Design review of the part built by this model. Coordinates are the model's own, in mm. Face numbers are marked on the shaded views. A direction names the side the tool comes from. Give positions to 0.01 mm unless a question says otherwise; leave off trailing zeros. Write each loop counter-clockwise with the first axis right and the second up, starting at its lowest first coordinate (ties: lowest second). Pieces come first, ordered by that corner, then holes. Notation, with made-up numbers: M 78,-21.5 L 129,-21.5 A4 ccw 129,-16.5 Z; hole C 76.5,-6 d7. An arc over 180 degrees is marked long. Answer in a Markdown table with one row per item.
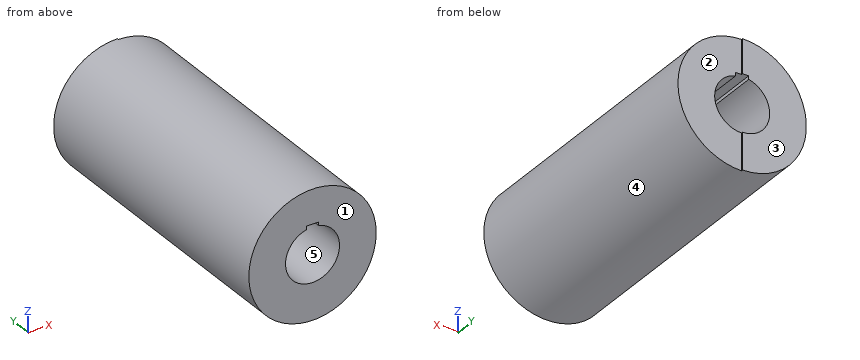
```python
from build123d import *

# Parameters (mm, degrees)
F1_R     = 210
F1_R_2   = 89
F2_DEPTH = 960
F3_W     = 40
F3_H     = 35.969428
F4_DEPTH = 1035
F6_DEPTH = 5


with BuildPart() as f2:
    # F1 (on face) → F2 (new body)
    with BuildSketch(Plane.XZ):
        Circle(F1_R)
        Circle(F1_R_2, mode=Mode.SUBTRACT)
    extrude(amount=F2_DEPTH)

    # F3 (on face) → F4 (cut)
    with BuildSketch(Plane.XZ.offset(960)):
        with Locations((0, 80.015286)):
            Rectangle(F3_W, F3_H)
    extrude(amount=-F4_DEPTH, mode=Mode.SUBTRACT)

    # F5 (on face) → F6 (cut)
    with BuildSketch(Plane.XZ):
        Polygon((0, 269.126058), (0, 0), (0, -241.775826), (255.997956, -190.357447), (264.750004, 22.974176), (219.895661, 219.895661), (88.614672, 269.126058), align=None)
    extrude(amount=F6_DEPTH, mode=Mode.SUBTRACT)


solid = f2.part
```
1) Add section B-B (y = -860). Write out the cut boundary in (x, z), and give its area (3 significant figures).
Geometry says:
| item | result |
|---|---|
| outline | C 0,0 d420; hole M -20,86.72 A89 ccw long 20,86.72 L 20,98 L -20,98 Z |
| area | 113,000 mm^2 |
2) Insertion check: P1, Ø2, axis at y = -452.5, z = 120.5, coming from the -X side; P2, Ø1.5, axis at y = -2, z = -179, coming from the +X side; P3, Ø5, axis at x = 155, y = -710, coming from the +Z side. Each pin has a flat end and moves straight along its axis. Give the tip position at first contact, or say it passes through.
Geometry says:
| item | result |
|---|---|
| P1 | x = -172.68 |
| P2 | x = 0 |
| P3 | z = 144.37 |
3) The part is to be moulded in two halves that separate along Z. For the marked faces 3, 4 and 5, say which applies: released by +Z, released by -Z, zero draft, split by the parting line, or undercut.
Geometry says:
| item | result |
|---|---|
| face 3 | zero draft |
| face 4 | split by the parting line |
| face 5 | undercut |
4) Add section C-C (x = -47.5). Write out the cut boundary in (y, z).
Geometry says:
| item | result |
|---|---|
| outline | M -960,-204.56 L 0,-204.56 L 0,-75.26 L -960,-75.26 Z; M -960,75.26 L 0,75.26 L 0,204.56 L -960,204.56 Z |
5) For the marked faces 1 and 2, list the 3-axis set-ups (+Z, -Z, +X, -X, +Y, -Y) from which the entire face can be reached by the end or side of a thin tool; tool diameter is ignored.
Geometry says:
| item | result |
|---|---|
| face 1 | +Z, -Z, +X, -X, -Y |
| face 2 | +Z, -Z, +X, +Y |
6) To check wall thickness, follow probe 1 along X at (y, z) = (-320, 6); probe 2 along X at (y, z) = (-471, 0); probe 3 along Z at (x, y) = (0, -335). State the ranges of each line that lie inside material, in increasing order. Write a range as [from, to].
Geometry says:
| item | result |
|---|---|
| probe 1 | [-209.91, -88.8], [88.8, 209.91] |
| probe 2 | [-210, -89], [89, 210] |
| probe 3 | [-210, -89], [98, 210] |
7) Add section D-D (z = -175). Write out the cut boundary in (x, y), and give its area (3 significant figures).
Geometry says:
| item | result |
|---|---|
| outline | M -116.08,-960 L 116.08,-960 L 116.08,-5 L 0,-5 L 0,0 L -116.08,0 Z |
| area | 222,000 mm^2 |
8) Add section A-A (z = 0). Write out the cut boundary in (x, y), and give its area (3 significant figures).
Geometry says:
| item | result |
|---|---|
| outline | M -210,-960 L -89,-960 L -89,0 L -210,0 Z; M 89,-960 L 210,-960 L 210,-5 L 89,-5 Z |
| area | 232,000 mm^2 |
